Design review of the part built by this model. Coordinates are the model's own, in mm. Face numbers are marked on the shaded views. Coordinates: 2 decimals unless noted, no trailing zeros. Loops run counter-clockwise (first coordinate to the right, second up) from the corner with the lowest first, then second, coordinate; pieces in that order, holes last. Notation, with made-up numbers: M 66,-9 L 112,-9 A15 cw 112,7 Z; hole C 62.25,-9 d2. An arc over 180 degrees is marked long. One line per item, written item: value.
```python
from build123d import *

# Parameters (mm, degrees)
F1_DEPTH = 12
F2_R     = 5.08
F3_R     = 5.08


with BuildPart() as f1:
    # F0 (on Front) → F1 (new body)
    with BuildSketch(Plane.XZ):
        with BuildLine():
            ThreePointArc((-19.800265, 0), (0, 19.800265), (19.800265, 0))
            Line((19.800265, 0), (31.800265, 0))
            Line((31.800265, 0), (31.800265, 10))
            ThreePointArc((31.800265, 10), (0, 28.488275), (-31.800265, 10))
            Line((-31.800265, 10), (-31.800265, 0))
            Line((-31.800265, 0), (-19.800265, 0))
        make_face()
    extrude(amount=F1_DEPTH)

    # F2
    f2_edges = [f1.edges().sort_by_distance(p)[0] for p in [
        (31.800265, -6, 10),
        (31.800265, -6, 0),
        (-31.800265, -6, 10),
        (-31.800265, -6, 0),
    ]]
    fillet(f2_edges, radius=F2_R)

    # F3
    f3_edges = [f1.edges().sort_by_distance(p)[0] for p in [
        (19.800265, -6, 0),
        (-19.800265, -6, 0),
    ]]
    fillet(f3_edges, radius=F3_R)


solid = f1.part
```
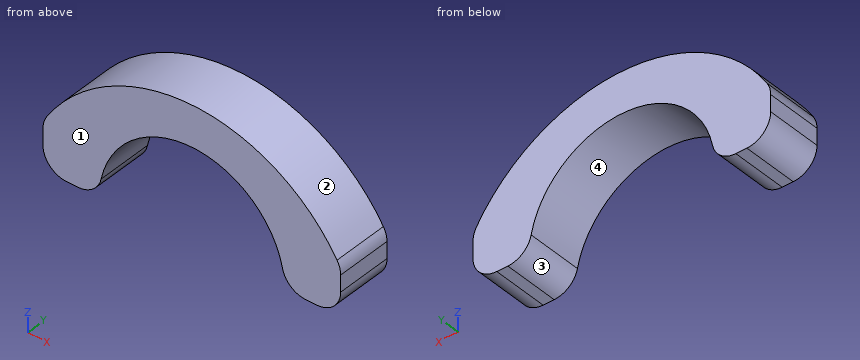
(1) We need section C-C on x = -14.5. State the section outline as (y, z) points.
Reply:
outline: M -12,13.48 L 0,13.48 L 0,25.49 L -12,25.49 Z
(2) We need section D-D on z = 17.75. State the section outline as (x, y) points.
Reply:
outline: M -25.9,-12 L -8.77,-12 L -8.77,0 L -25.9,0 Z; M 8.77,-12 L 25.9,-12 L 25.9,0 L 8.77,0 Z
(3) We need section B-B on y = -5.75. State the section outline as (x, z) points, then the cut area to 3 significant figures.
Reply:
outline: M -31.8,5.08 A5.08 ccw -26.72,0 L -24.36,0 A5.08 ccw -19.38,4.04 A19.8 cw 19.38,4.04 A5.08 ccw 24.36,0 L 26.72,0 A5.08 ccw 31.8,5.08 L 31.8,8.6 A5.08 ccw 31.03,11.29 A36.59 ccw -31.03,11.29 A5.08 ccw -31.8,8.6 Z
area: 835 mm2
(4) We need section A-A on z = 2.75. State the section outline as (x, y) points, then the cut area to 3 significant figures.
Reply:
outline: M -31.23,-12 L -19.84,-12 L -19.84,0 L -31.23,0 Z; M 19.84,-12 L 31.23,-12 L 31.23,0 L 19.84,0 Z
area: 273 mm2
(5) Mouldability with a two-part tool opening along X and no side actions: class the marked faces 1, 2, 3 and 4 as released by +X, released by -X, zero draft, split by the parting line, or undercut.
Reply:
face 1: zero draft
face 2: split by the parting line
face 3: undercut
face 4: undercut
(6) To check wall thickness, follow line 1 along X through (y, z) = (-4.75, 17.5); line 2 along X through (y, z) = (-4.5, 6.25); line 3 along Z through (x, y) = (5.5, -1.75). State the ranges of each line that lie inside material, in increasing order. Write a range as [from, to].
Reply:
line 1: x = [-26.14, -9.26], [9.26, 26.14]
line 2: x = [-31.8, -18.79], [18.79, 31.8]
line 3: z = [19.02, 28.07]
(7) Insertion check: pin 1 (1 mm diameter, centred on y = -6.5, z = 22, fed in from +X); pin 2 (5 mm diameter, centred on x = 21.5, y = -10.5, fed in from +Z); pin 3 (5 mm diameter, centred on x = 1, y = -9, fed in from -Z). Each pin has a flat end and moves straight along its axis. Give the tip position at first contact, or say it passes through.
Reply:
pin 1: stops at x = 21.51
pin 2: stops at z = 23.17
pin 3: stops at z = 19.49
